Model file for the job. Use its own axes, mm. Face numbers are marked on the shaded views. A direction names the side the tool comes from. Give positions to 0.01 mm unless a question says otherwise; leave off trailing zeros. Loops run counter-clockwise (first coordinate to the right, second up) from the corner with the lowest first, then second, coordinate; pieces in that order, holes last. Notation, with made-up numbers: M -29.5,58 L 28.5,58 A31 ccw 28.5,84 Z; hole C 88,12 d11. An arc over 180 degrees is marked long. Use CSV: the item, a comma, the result in double quotes. Start each with the question number.
(1) Slice it at C-C on z = 1512.5. List the corners of the cut face in (x, y).
(2) Two-plate mould, pull along Y, no slides. Class the marked faces 1 and 2: pulls with the +Y half, pulls with the -Y half, needs draft (parallel to the pull), parting line crosses it, or undercut.
(3) Wall check: line 1 along Z through (x, y) = (93, -83). Give the ranges that are in metal, low to high. Write a range as from..to.
(4) Tool access for the marked faces 3, 4, 5 and 6: list every direction of +Z, -Z, +X, -X, +Y, -Y with a clear straight run to the whole face (end or side of a thin tool).
(5) Slice it at A-A on x = 211.5. State how many separate pieces and enclosed holes the cut face has, and give its area (3 significant figures).
```python
from build123d import *

# Parameters (mm, degrees)
F0_W     = 609.6
F0_H     = 1219.2
F1_DEPTH = 1828.8
F2_W     = 1168.4
F2_H     = 381
F3_DEPTH = 609.601
F4_W     = 558.8
F4_H     = 381
F5_DEPTH = 1219.201


with BuildPart() as f1:
    # F0 (on Top) → F1 (new body)
    with BuildSketch(Plane.XY):
        Rectangle(F0_W, F0_H)
    extrude(amount=F1_DEPTH)

    # F2 (on face) → F3 (cut, through all)
    with BuildSketch(Plane.YZ.offset(304.8)):
        with Locations((0, 215.9)):
            Rectangle(F2_W, F2_H)
        with Locations((0, 671.647025)):
            Rectangle(F2_W, F2_H)
        with Locations((0, 1127.394051)):
            Rectangle(F2_W, F2_H)
        with Locations((0, 1583.141076)):
            Rectangle(F2_W, F2_H)
    extrude(amount=-F3_DEPTH, mode=Mode.SUBTRACT)

    # F4 (on face) → F5 (cut, through all)
    with BuildSketch(Plane.XZ.offset(609.6)):
        with Locations((0, 215.9)):
            Rectangle(F4_W, F4_H)
        with Locations((0, 670.56)):
            Rectangle(F4_W, F4_H)
        with Locations((0, 1125.22)):
            Rectangle(F4_W, F4_H)
        with Locations((0, 1579.88)):
            Rectangle(F4_W, F4_H)
    extrude(amount=-F5_DEPTH, mode=Mode.SUBTRACT)


solid = f1.part
```
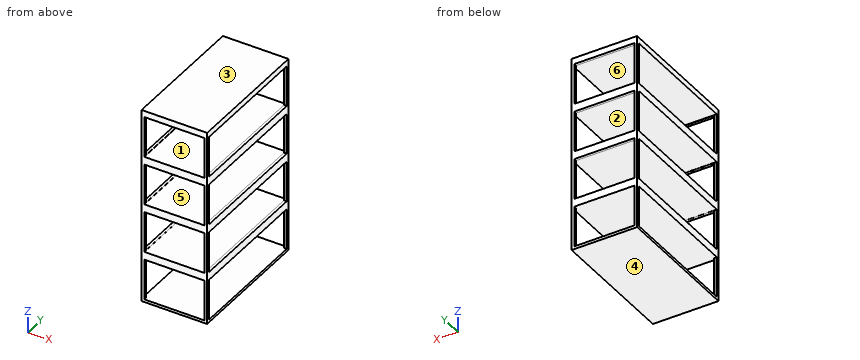
Reply:
1,outline,"M -304.8,-609.6 L -279.4,-609.6 L -279.4,-584.2 L -304.8,-584.2 Z; M -304.8,584.2 L -279.4,584.2 L -279.4,609.6 L -304.8,609.6 Z; M 279.4,-609.6 L 304.8,-609.6 L 304.8,-584.2 L 279.4,-584.2 Z; M 279.4,584.2 L 304.8,584.2 L 304.8,609.6 L 279.4,609.6 Z"
2,face 1,"needs draft"
2,face 2,"undercut"
3,line 1,"z = 0..25.4, 406.4..480.06, 862.15..934.72, 1317.89..1389.38, 1773.64..1828.8"
4,face 3,"+Z, +X, -X, +Y, -Y"
4,face 4,"-Z, +X, -X, +Y, -Y"
4,face 5,"+Y, -Y"
4,face 6,"+X, -X"
5,separate pieces,"5"
5,enclosed holes,"0"
5,area,"364,000 mm^2"
